Check sheet for the drawn part. Datum: minimum x, y, z corner. Units: mm. A direction names the side the tool comes from. Give positions to 0.01 mm unless a question says otherwise; leave off trailing zeros. Order: outer loops, then holes, each group sorted by start corner. A loop starts at its lowest first (then second) coordinate and runs counter-clockwise, first axis right, second up.
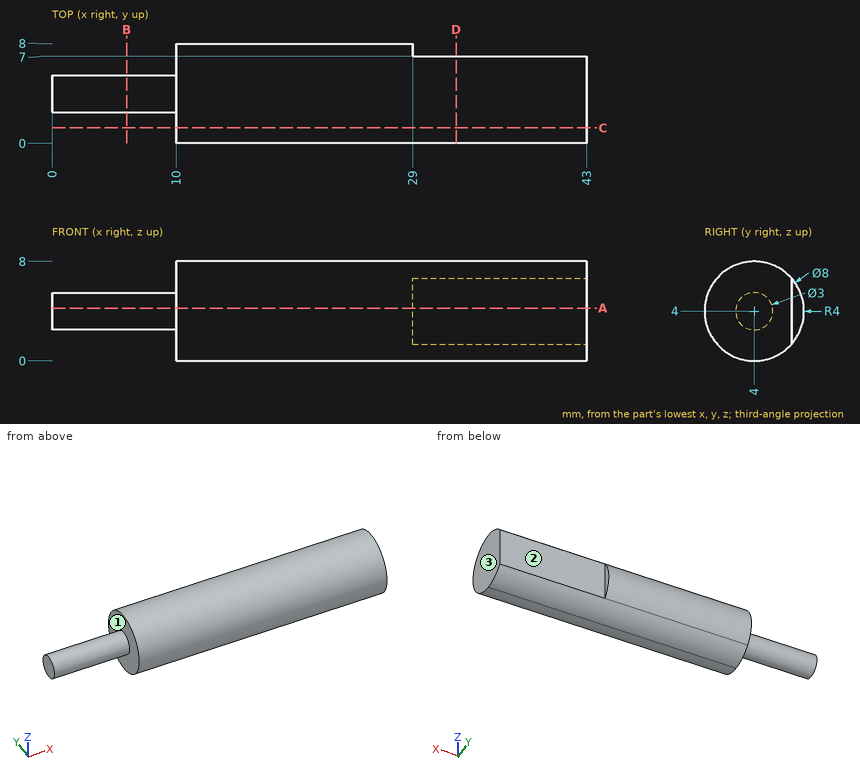
(1) Section check B-B, the plane x = 6. Enter the section's corners in (y, z), then the cut area to 3 significant figures.
Solved:
outline: circle Ø3 at (4, 4)
area: 7.07 mm2
(2) Set-up check for the marked faces 1, 2 and 3: record each of +Z, -Z, +X, -X, +Y, -Y from which the full face is reachable in a straight line by a thin tool's end or side.
Solved:
face 1: -X
face 2: +Z, -Z, +X, +Y
face 3: +Z, -Z, +X, +Y, -Y
(3) Section check A-A, the plane z = 4.25. Enter the section's corners in (x, y).
Solved:
outline: (0, 2.52) - (10, 2.52) - (10, 0.01) - (43, 0.01) - (43, 7) - (29, 7) - (29, 7.99) - (10, 7.99) - (10, 5.48) - (0, 5.48) - close
(4) Section check C-C, the plane y = 1.25. Enter the section's corners in (x, z).
Solved:
outline: (10, 1.1) - (43, 1.1) - (43, 6.9) - (10, 6.9) - close
(5) Section check D-D, the plane x = 32.5. Enter the section's corners in (y, z).
Solved:
outline: (7, 1.35) - (7, 6.65) arc R4 ccw (long way) to start
(6) Scan lines: line 1 (Z direction, x = 20, y = 3.75); line 2 (X direction, y = 2.75, z = 2); line 3 (X direction, y = 7.25, z = 5.5). Record each from-to range of solid material in increasing order.
Solved:
line 1: z = 0.01 to 7.99
line 2: x = 10 to 43
line 3: x = 10 to 29
(7) Go/stop test with flat-tipped pins: pin 1 (4 mm diameter, centred on x = 34.5, z = 5, fed in from +Y); pin 2 (3 mm diameter, centred on x = 36, z = 1, fed in from -Y); pin 3 (3 mm diameter, centred on y = 1, z = 3, fed in from -X). Record where each tip stops, or that it passes through.
Solved:
pin 1: stops at y = 7
pin 2: stops at y = 0.29
pin 3: stops at x = 10
